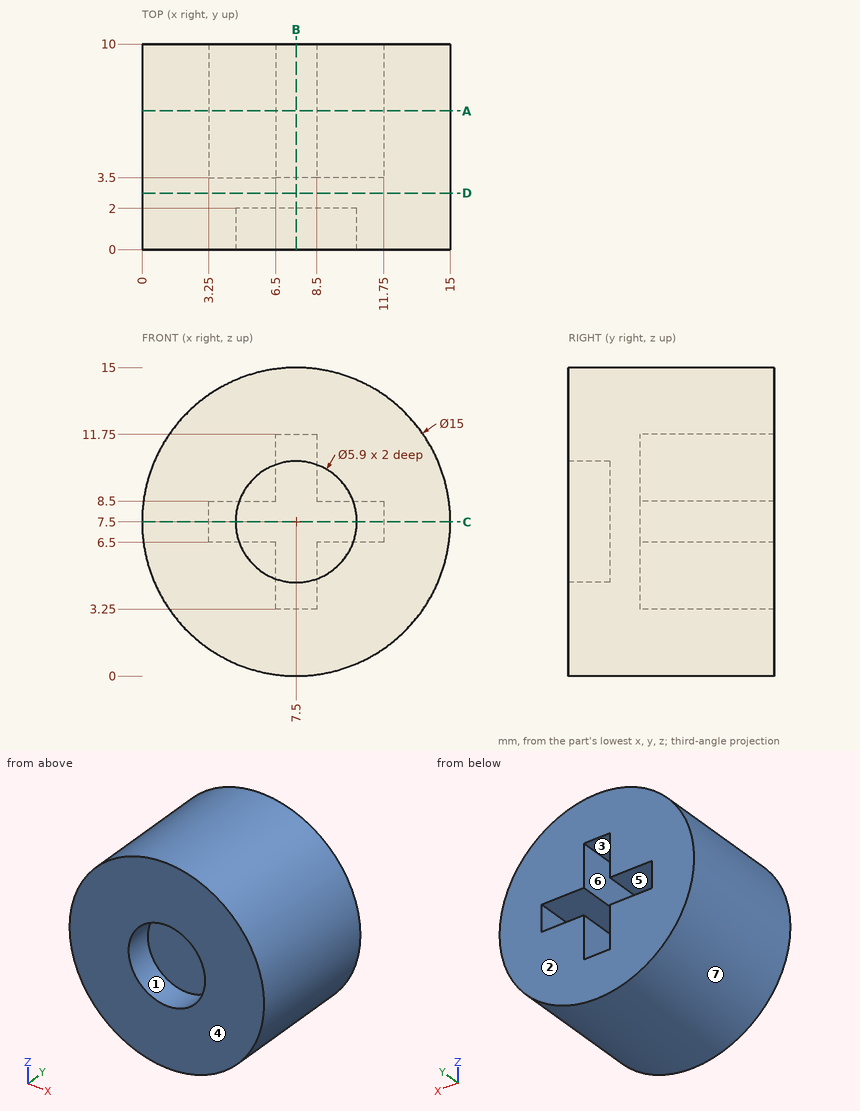
Part print with two shaded views. Sizes in mm from the minimum x, y, z corner. A direction names the side the tool comes from. Give positions to 0.01 mm unless a question says otherwise; leave off trailing zeros. Order: outer loops, then holes, each group sorted by start corner. A loop starts at its lowest first (then second) coordinate and runs counter-clockwise, first axis right, second up.
(1) Mould opens along X. For the marked faces 4, 5, 6 and 7 say: released by +X, released by -X, zero draft, split by the parting line, or undercut.
(2) Saw through at C-C, the plane z = 7.5. Give the cut face in (x, y).
(3) Saw through at A-A, the plane y = 6.75. Give the cut face in (x, z).
(4) Drill centre lines: L1, parallel to Z at x = 7.5, y = 1.4; L2, parallel to Z at x = 10.75, y = 7; L3, parallel to X at y = 8.25, z = 8.25. Where is each one in solid material? Low to high.
(5) Saw through at B-B, the plane x = 7.5. Give the cut face in (y, z), then the cut area to 4 significant figures.
(6) Saw through at D-D, the plane y = 2.75. Give the cut face in (x, z), then the cut area to 3 significant figures.
(7) Flat gauge pins, fed straight in: pin 1 (3.5 mm diameter, centred on y = 8, z = 5, fed in from +X); pin 2 (1.5 mm diameter, centred on y = 5, z = 2.5, fed in from -X); pin 3 (2 mm diameter, centred on y = 6.5, z = 12, fed in from +X). Where does each tip first touch, or does it go through?
(8) Tool access for the marked faces 1, 2 and 3: list every direction of +Z, -Z, +X, -X, +Y, -Y with a clear straight run to the whole face (end or side of a thin tool).
Results found:
1. face 4: zero draft
1. face 5: undercut
1. face 6: undercut
1. face 7: split by the parting line
2. outline: (0, 0) - (4.55, 0) - (4.55, 2) - (10.45, 2) - (10.45, 0) - (15, 0) - (15, 10) - (11.75, 10) - (11.75, 3.5) - (3.25, 3.5) - (3.25, 10) - (0, 10) - close
3. outline: circle Ø15 at (7.5, 7.5); hole (3.25, 6.5) - (6.5, 6.5) - (6.5, 3.25) - (8.5, 3.25) - (8.5, 6.5) - (11.75, 6.5) - (11.75, 8.5) - (8.5, 8.5) - (8.5, 11.75) - (6.5, 11.75) - (6.5, 8.5) - (3.25, 8.5) - close
4. L1: z = 0 to 4.55, 10.45 to 15
4. L2: z = 0.74 to 6.5, 8.5 to 14.26
4. L3: x = 0.04 to 3.25, 11.75 to 14.96
5. outline: (0, 0) - (10, 0) - (10, 3.25) - (3.5, 3.25) - (3.5, 11.75) - (10, 11.75) - (10, 15) - (0, 15) - (0, 10.45) - (2, 10.45) - (2, 4.55) - (0, 4.55) - close
5. area: 82.95 mm2
6. outline: circle Ø15 at (7.5, 7.5)
6. area: 177 mm2
7. pin 1: stops at x = 14.96
7. pin 2: stops at x = 1.32
7. pin 3: stops at x = 14.13
8. face 1: -Y
8. face 2: +Z, -Z, +X, -X, +Y
8. face 3: +Y
